from build123d import *

# Parameters (mm, degrees)
SKETCH1_R           = 2.5
SKETCH1_W           = 15
SKETCH1_H           = 40
BOSS_EXTRUDE1_DEPTH = 9.7
BOSS_EXTRUDE2_START = -5
SKETCH2_R           = 2.38
BOSS_EXTRUDE2_DEPTH = 10
FILLET1_R           = 1
FILLET2_R           = 6


with BuildPart() as part:
    # Sketch1 → Boss-Extrude1 (new body)
    # profile 1 of 2: a face of its own
    with BuildSketch(Plane.XY):
        with BuildLine():
            ThreePointArc((-17.5, 50), (0, 67.5), (17.5, 50))
            Line((17.5, 50), (17.5, -50))
            Line((17.5, -50), (-17.5, -50))
            Line((-17.5, -50), (-17.5, 50))
        make_face()
        with Locations((0, -40)):
            Circle(SKETCH1_R, mode=Mode.SUBTRACT)
        Rectangle(SKETCH1_W, SKETCH1_H, mode=Mode.SUBTRACT)
    # profile 2 of 2: a face of its own
    with BuildSketch(Plane.XY):
        with BuildLine():
            ThreePointArc((-17.5, 50), (0, 67.5), (17.5, 50))
            Line((17.5, 50), (-17.5, 50))
        make_face()
    extrude(amount=BOSS_EXTRUDE1_DEPTH)

    # Sketch2 → Boss-Extrude2 (add, symmetric)
    with BuildSketch(Plane.XY.offset(9.7).offset(BOSS_EXTRUDE2_START)):
        with Locations((0, 62)):
            Circle(SKETCH2_R)
    extrude(amount=BOSS_EXTRUDE2_DEPTH, both=True)

    # Fillet1
    fillet1_edges = [part.edges().sort_by_distance(p)[0] for p in [
        (-2.38, 62, -5.3),
        (-2.38, 62, 14.7),
    ]]
    fillet(fillet1_edges, radius=FILLET1_R)

    # Fillet2
    # the kernel refuses this fillet: 6 mm, written as the material it takes off along each edge
    with BuildSketch(Plane(origin=(7.5, 20, 0), x_dir=(1, 0, 0), z_dir=(0, -1, 0)), Plane(origin=(7.5, 20, 9.7), x_dir=(0, 0, -1), z_dir=(0, -1, 0)), Plane(origin=(-7.5, -20, 0), x_dir=(-1, 0, 0), z_dir=(0, 1, 0)), Plane(origin=(-7.5, -20, 9.7), x_dir=(0, 0, -1), z_dir=(0, 1, 0))) as fillet2_piece_1:
        with BuildLine():
            CenterArc((FILLET2_R, FILLET2_R), FILLET2_R, 180, 90)
            Line((0, FILLET2_R), (0, 0))
            Line((0, 0), (FILLET2_R, 0))
        make_face()
    extrude(amount=40, mode=Mode.SUBTRACT)


solid = part.part
Geometry: final body of the model. Coordinates: model frame, mm. A direction names the side the tool comes from. Round coordinates to 2 decimals unless told otherwise and drop trailing zeros. Loops run counter-clockwise (first coordinate to the right, second up) from the corner with the lowest first, then second, coordinate; pieces in that order, holes last. Notation, with made-up numbers: M -18.75,50.5 L 8.25,50.5 A20 cw 8.25,70.5 Z; hole C 61,36.5 d2. An arc over 180 degrees is marked long. One line per question, with ' | ' between items.
(1) Access query for faces 5 (the flat face through (17.5, 1, 5)), 6 (the cylindrical face through (-0.516, 59.677, -2.12)), 7 (the cylindrical face through (-9.73, -0.28, 8.37)). Directions: +Z, -Z, +X, -X, +Y, -Y. A direction counts if a zero-diameter tool reaches every point of the face in a straight line with its end or side. Return the directions, or none.
Check result:
face 5: +Z, -Z, +X, +Y, -Y | face 6: -Z | face 7: +Z
(2) Cut plane A-A on y = -40. Return the cut outline in (x, z).
Check result:
outline: M -17.5,0 L -2.5,0 L -2.5,9.7 L -17.5,9.7 Z; M 2.5,0 L 17.5,0 L 17.5,9.7 L 2.5,9.7 Z
(3) Material intervals for line 1 along Y through (x, z) = (0, 5); line 2 along Y through (x, z) = (-0.5, 3.75); line 3 along Y through (x, z) = (10, 0.25), sorted ascending. Write a range as from..to.
Check result:
line 1: y = -50..-42.5, -37.5..-20, 20..67.5 | line 2: y = -50..-42.45, -37.55..-20, 20..67.49 | line 3: y = -50..-20, 20..64.36
(4) Cut plane C-C on z = 2. Return the cut outline in (x, y), plus the area to 3 significant figures.
Check result:
outline: M -17.5,-50 L 17.5,-50 L 17.5,50 A17.5 ccw -17.5,50 Z; hole M -9.03,-20 L 9.03,-20 L 9.03,20 L -9.03,20 Z; hole C 0,-40 d5 | area: 3,240 mm2
(5) Cut plane D-D on x = 5. Return the cut outline in (y, z), plus the area to 3 significant figures.
Check result:
outline: M -50,0 L -20,0 L -20,9.7 L -50,9.7 Z; M 20,0 L 66.77,0 L 66.77,9.7 L 20,9.7 Z | area: 745 mm2
(6) Cut plane B-B on x = 0. Return the cut outline in (y, z), plus the area to 3 significant figures.
Check result:
outline: M -50,0 L -42.5,0 L -42.5,9.7 L -50,9.7 Z; M -37.5,0 L -20,0 L -20,9.7 L -37.5,9.7 Z; M 20,0 L 59.62,0 L 59.62,-4.3 A1 ccw 60.62,-5.3 L 63.38,-5.3 A1 ccw 64.38,-4.3 L 64.38,0 L 67.5,0 L 67.5,9.7 L 64.38,9.7 L 64.38,13.7 A1 ccw 63.38,14.7 L 60.62,14.7 A1 ccw 59.62,13.7 L 59.62,9.7 L 20,9.7 Z | area: 751 mm2
(7) Pull-direction query (X, two-part tool) for faces 1 (the cylindrical face through (9.73, 0.28, 8.37)), 2 (the cylindrical face through (-0.516, 59.677, 11.728)), 3 (the cylindrical face through (-0.54, -42.44, 4.78)), 4 (the flat face through (0, -50, 5)); classes: +X half, -X half, draft (parallel to the pull), parting line (faces both ways), or undercut.
Check result:
face 1: undercut | face 2: parting line | face 3: undercut | face 4: draft
(8) Contact query for flat-ended pins moving along their axis: P1, Ø3, axis at x = -11.5, y = 30.5, coming from the -Z side; P2, Ø17.5, axis at x = -6.5, y = -11, coming from the +Z side; P3, Ø1, axis at x = 6.5, z = 3.5, coming from the +Y side. Output: stop coordinate, or through.
Check result:
P1: stops at z = 0 | P2: stops at z = 9.7 | P3: stops at y = 66.44
